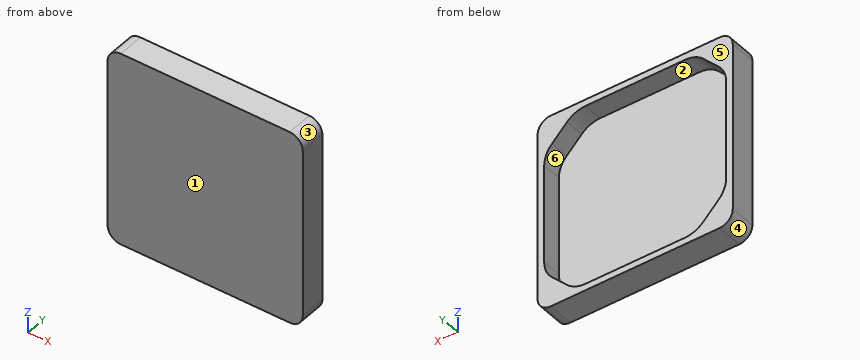
Autodesk Inventor part; units mm, degrees
ref_plane "YZ Plane" through (0, 0, 0) normal (1, 0, 0) x (0, 1, 0)
ref_plane "XZ Plane" through (0, 0, 0) normal (0, 1, 0) x (-1, 0, 0)
ref_plane "XY Plane" through (0, 0, 0) normal (0, 0, 1) x (1, 0, 0)
sketch "Sketch1" plane through (0, 0, 0) normal (0, 1, 0) x (-1, 0, 0)
  circle A0 centre (0, 0) radius 18.3769
  line L0 (18.3769, 18.3769) -> (-18.3769, -18.3769) construction
  line L1 (-18.3769, 18.3769) -> (18.3769, -18.3769) construction
  line L2 (13.335, 21.59) -> (-13.335, 21.59)
  line L3 (-21.59, 13.335) -> (-21.59, -13.335)
  line L4 (-13.335, -21.59) -> (13.335, -21.59)
  line L5 (21.59, -13.335) -> (21.59, 13.335)
  line L6 (21.59, 21.59) -> (-21.59, -21.59) construction
  line L7 (-21.59, 21.59) -> (21.59, -21.59) construction
  line L8 (21.59, 13.335) -> (13.335, 21.59)
  line L9 (-13.335, 21.59) -> (-21.59, 13.335)
  line L10 (-21.59, -13.335) -> (-13.335, -21.59)
  line L11 (13.335, -21.59) -> (21.59, -13.335)
  circle A1 centre (15.24, -15.24) radius 1.0033
  circle A2 centre (-15.24, -15.24) radius 1.0033
  circle A3 centre (-15.24, 15.24) radius 1.0033
  circle A4 centre (15.24, 15.24) radius 1.0033
  line L12 (11.9917, -21.9869) -> (-11.9917, -21.9869)
  line L13 (-21.9869, -11.9917) -> (-21.9869, 11.9917)
  line L14 (-11.9917, 21.9869) -> (11.9917, 21.9869)
  line L15 (21.9869, 11.9917) -> (21.9869, -11.9917)
  line L16 (-20.3962, 23.5712) -> (20.3962, 23.5712)
  line L17 (23.5712, 20.3962) -> (23.5712, -20.3962)
  line L18 (20.3962, -23.5712) -> (-20.3962, -23.5712)
  line L19 (-23.5712, -20.3962) -> (-23.5712, 20.3962)
  line L20 (-23.5712, 23.5712) -> (23.5712, -23.5712) construction
  line L21 (23.5712, 23.5712) -> (-23.5712, -23.5712) construction
  arc A5 (20.3962, -23.5712) -> (23.5712, -20.3962) centre (20.3962, -20.3962) ccw
  arc A6 (-23.5712, -20.3962) -> (-20.3962, -23.5712) centre (-20.3962, -20.3962) ccw
  arc A7 (-20.3962, 23.5712) -> (-23.5712, 20.3962) centre (-20.3962, 20.3962) ccw
  arc A8 (23.5712, 20.3962) -> (20.3962, 23.5712) centre (20.3962, 20.3962) ccw
  circle A9 centre (20.3962, -20.3962) radius 1.0033
  circle A10 centre (-20.3962, -20.3962) radius 1.0033
  circle A11 centre (-20.3962, 20.3962) radius 1.0033
  circle A12 centre (20.3962, 20.3962) radius 1.0033
  line L22 (16.4818, -20.127) -> (20.127, -16.4818)
  line L23 (20.127, 16.4818) -> (16.4818, 20.127)
  line L24 (-16.4818, 20.127) -> (-20.127, 16.4818)
  line L25 (-20.127, -16.4818) -> (-16.4818, -20.127)
  arc A13 (21.9869, 11.9917) -> (20.127, 16.4818) centre (15.6369, 11.9917) ccw
  arc A14 (16.4818, 20.127) -> (11.9917, 21.9869) centre (11.9917, 15.6369) ccw
  arc A15 (-11.9917, 21.9869) -> (-16.4818, 20.127) centre (-11.9917, 15.6369) ccw
  arc A16 (-20.127, 16.4818) -> (-21.9869, 11.9917) centre (-15.6369, 11.9917) ccw
  arc A17 (-21.9869, -11.9917) -> (-20.127, -16.4818) centre (-15.6369, -11.9917) ccw
  arc A18 (-16.4818, -20.127) -> (-11.9917, -21.9869) centre (-11.9917, -15.6369) ccw
  arc A19 (11.9917, -21.9869) -> (16.4818, -20.127) centre (11.9917, -15.6369) ccw
  arc A20 (20.127, -16.4818) -> (21.9869, -11.9917) centre (15.6369, -11.9917) ccw
  line L26 (4.3815, -5.969) -> (4.3815, -12.5476)
  line L27 (2.794, -14.1351) -> (-2.794, -14.1351)
  line L28 (-4.3815, -12.5476) -> (-4.3815, -5.969)
  line L29 (4.3815, 5.969) -> (4.3815, 12.5476)
  line L30 (2.794, 14.1351) -> (-2.794, 14.1351)
  line L31 (-4.3815, 12.5476) -> (-4.3815, 5.969)
  line L32 (-5.969, -4.3815) -> (-12.5476, -4.3815)
  line L33 (-14.1351, -2.794) -> (-14.1351, 2.794)
  line L34 (-12.5476, 4.3815) -> (-5.969, 4.3815)
  line L35 (5.969, -4.3815) -> (12.5476, -4.3815)
  line L36 (14.1351, -2.794) -> (14.1351, 2.794)
  line L37 (12.5476, 4.3815) -> (5.969, 4.3815)
  arc A21 (2.794, -14.1351) -> (4.3815, -12.5476) centre (2.794, -12.5476) ccw
  arc A22 (-4.3815, -12.5476) -> (-2.794, -14.1351) centre (-2.794, -12.5476) ccw
  arc A23 (-4.3815, -5.969) -> (-5.969, -4.3815) centre (-5.969, -5.969) ccw
  arc A24 (-14.1351, -2.794) -> (-12.5476, -4.3815) centre (-12.5476, -2.794) ccw
  arc A25 (-14.1351, -2.794) -> (-12.5476, -4.3815) centre (-12.5476, -2.794) ccw
  arc A26 (-12.5476, 4.3815) -> (-14.1351, 2.794) centre (-12.5476, 2.794) ccw
  arc A27 (-5.969, 4.3815) -> (-4.3815, 5.969) centre (-5.969, 5.969) ccw
  arc A28 (-2.794, 14.1351) -> (-4.3815, 12.5476) centre (-2.794, 12.5476) ccw
  arc A29 (4.3815, 12.5476) -> (2.794, 14.1351) centre (2.794, 12.5476) ccw
  arc A30 (4.3815, 5.969) -> (5.969, 4.3815) centre (5.969, 5.969) ccw
  arc A31 (14.1351, 2.794) -> (12.5476, 4.3815) centre (12.5476, 2.794) ccw
  arc A32 (12.5476, -4.3815) -> (14.1351, -2.794) centre (12.5476, -2.794) ccw
  arc A33 (5.969, -4.3815) -> (4.3815, -5.969) centre (5.969, -5.969) ccw
  line L38 (-2.794, -14.9289) -> (2.794, -14.9289)
  arc A34 (2.794, -14.9289) -> (5.1753, -12.5476) centre (2.794, -12.5476) ccw
  line L39 (5.1753, -12.5476) -> (5.1753, -5.969)
  arc A35 (5.969, -5.1753) -> (5.1753, -5.969) centre (5.969, -5.969) ccw
  line L40 (5.969, -5.1753) -> (12.5476, -5.1753)
  arc A36 (12.5476, -5.1753) -> (14.9289, -2.794) centre (12.5476, -2.794) ccw
  line L41 (14.9289, -2.794) -> (14.9289, 2.794)
  arc A37 (14.9289, 2.794) -> (12.5476, 5.1753) centre (12.5476, 2.794) ccw
  line L42 (12.5476, 5.1753) -> (5.969, 5.1753)
  arc A38 (5.1753, 5.969) -> (5.969, 5.1753) centre (5.969, 5.969) ccw
  line L43 (5.1753, 5.969) -> (5.1753, 12.5476)
  arc A39 (5.1753, 12.5476) -> (2.794, 14.9289) centre (2.794, 12.5476) ccw
  line L44 (2.794, 14.9289) -> (-2.794, 14.9289)
  arc A40 (-2.794, 14.9289) -> (-5.1753, 12.5476) centre (-2.794, 12.5476) ccw
  line L45 (-5.1753, 12.5476) -> (-5.1753, 5.969)
  arc A41 (-5.969, 5.1753) -> (-5.1753, 5.969) centre (-5.969, 5.969) ccw
  line L46 (-5.969, 5.1753) -> (-12.5476, 5.1753)
  arc A42 (-12.5476, 5.1753) -> (-14.9289, 2.794) centre (-12.5476, 2.794) ccw
  line L47 (-14.9289, 2.794) -> (-14.9289, -2.794)
  arc A43 (-14.9289, -2.794) -> (-12.5476, -5.1753) centre (-12.5476, -2.794) ccw
  line L48 (-12.5476, -5.1753) -> (-5.969, -5.1753)
  arc A44 (-5.1753, -5.969) -> (-5.969, -5.1753) centre (-5.969, -5.969) ccw
  line L49 (-5.1753, -5.969) -> (-5.1753, -12.5476)
  arc A45 (-5.1753, -12.5476) -> (-2.794, -14.9289) centre (-2.794, -12.5476) ccw
  point P0 (4.3815, -14.1351)
  point P1 (-4.3815, -14.1351)
  point P2 (4.3815, 14.1351)
  point P3 (-14.1351, 4.3815)
  point P4 (-4.3815, 4.3815)
  point P5 (14.1351, 4.3815)
  point P6 (4.3815, 4.3815)
  dimension "d33" = 36.7538
  dimension "d34" = 43.18
  dimension "d35" = 43.18
  dimension "d48" = 2.0066
  dimension "d49" = 2.0066
  dimension "d50" = 2.0066
  dimension "d51" = 2.0066
  dimension "d52" = 0.3969
  dimension "d53" = 47.1424
  dimension "d54" = 47.1424
  dimension "d55" = 3.175
  dimension "d56" = 2.0066
  dimension "d57" = 2.0066
  dimension "d58" = 2.0066
  dimension "d59" = 2.0066
  dimension "d62" = 6.35
  dimension "d79" = 8.763
  dimension "d84" = 1.5875
  dimension "d85" = 0.7937
  dimension "d86" = 9.7536
extrude "Extrusion9" add sketch "Sketch1" along normal blind 6.35 contours L16 A8 L17 A5 L18 A6 L19 A7 | A9 | A10 | A11 | A12
extrude "Extrusion10" add sketch "Sketch1" along normal blind 1.5875 contours A0 | L8 L5 L11 L4 L10 L3 L9 L2 | A1 | A2 | A3 | A4 | L12 A18 L25 A17 L13 A16 L24 A15 L14 A14 L23 A13 L15 A20 L22 A19 | L26 A21 L27 A22 L28 A23 L32 A24 L33 A26 L34 A27 L31 A28 L30 A29 L29 A30 L37 A31 L36 A32 L35 A33 | A45 L49 A44 L48 A43 L47 A42 L46 A41 L45 A40 L44 A39 L43 A38 L42 A37 L41 A36 L40 A35 L39 A34 L38
properties part number "SnakeControllerCase_v3"
The listing builds one solid part. Answer for the finished solid, in the listing's coordinates (mm). Face numbers are marked on the shaded views. A direction names the side the tool comes from. Coordinates: 2 decimals unless noted, no trailing zeros. Write each loop counter-clockwise with the first axis right and the second up, starting at its lowest first coordinate (ties: lowest second). Pieces come first, ordered by that corner, then holes. Notation, with made-up numbers: M -28,26 L -24,26 A24 ccw -24,51 Z; hole C 57.5,-27.75 d11. An arc over 180 degrees is marked long. Use a Markdown table: item, result. Add a question column.
1. Straight lines are drawn through the part: line 1 along X through (y, z) = (4.25, -10.5); line 2 along Y through (x, z) = (-7.5, -12.5). For each, find the intervals that lie inside material, in ascending order. Write a range as [from, to].
2. Section A-A (z = -7) is taken. Give the vertices of the cut face in (x, y), plus the area to 3 significant figures.
3. Which of the six approach directions +Z, -Z, +X, -X, +Y, -Y give full straight-line access (tool end or side, diameter ignored) to the marked faces 1 and 2?
4. Section B-B (x = -0.5) is taken. Give the vertices of the cut face in (y, z).
5. For a pull along X with two mould halves and no side action, classify the marked faces 3, 4, 5 and 6 as +X half, -X half, draft (parallel to the pull), parting line (faces both ways), or undercut.
6. Given P1, Ø22, axis at x = -4, z = 8.5, coming from the +Y side; P2, Ø4, axis at x = 9.5, z = -16, coming from the -Y side, each flat-ended and moving along its own axis, determine where each tip first touches the part or whether it passes through.
7. Section C-C (y = 3.25) is taken. Give the vertices of the cut face in (x, z) (3 decimals).
Data:
| question | item | result |
|---|---|---|
| 1 | line 1 | x = [-23.57, -21.99], [21.99, 23.57] |
| 1 | line 2 | y = [0, 1.59] |
| 2 | outline | M -23.57,0 L 23.57,0 L 23.57,6.35 L 21.99,6.35 L 21.99,1.59 L -21.99,1.59 L -21.99,6.35 L -23.57,6.35 Z |
| 2 | area | 89.9 mm2 |
| 3 | face 1 | +Z, -Z, +X, -X, -Y |
| 3 | face 2 | +Y |
| 4 | outline | M 0,-23.57 L 6.35,-23.57 L 6.35,-21.99 L 1.59,-21.99 L 1.59,21.99 L 6.35,21.99 L 6.35,23.57 L 0,23.57 Z |
| 5 | face 3 | +X half |
| 5 | face 4 | -X half |
| 5 | face 5 | draft |
| 5 | face 6 | undercut |
| 6 | P1 | stops at y = 1.59 |
| 6 | P2 | stops at y = 0 |
| 7 | outline | M -23.571,-20.396 A3.175 ccw -20.396,-23.571 L 20.396,-23.571 A3.175 ccw 23.571,-20.396 L 23.571,20.396 A3.175 ccw 20.396,23.571 L -20.396,23.571 A3.175 ccw -23.571,20.396 Z; hole M -21.987,-11.992 A6.35 ccw -20.127,-16.482 L -16.482,-20.127 A6.35 ccw -11.992,-21.987 L 11.992,-21.987 A6.35 ccw 16.482,-20.127 L 20.127,-16.482 A6.35 ccw 21.987,-11.992 L 21.987,11.992 A6.35 ccw 20.127,16.482 L 16.482,20.127 A6.35 ccw 11.992,21.987 L -11.992,21.987 A6.35 ccw -16.482,20.127 L -20.127,16.482 A6.35 ccw -21.987,11.992 Z |
